Read the model definition and answer for the solid it produces. Units are mm, in the model's axes. A direction names the side the tool comes from. Round coordinates to 2 decimals unless told otherwise and drop trailing zeros. Order: outer loops, then holes, each group sorted by start corner. A loop starts at its lowest first (then second) coordinate and runs counter-clockwise, first axis right, second up. Notation, with made-up numbers: (84.25, 16) - (97.25, 16) arc R26 cw to (97.25, 34) - close; hole circle Ø10 at (11.25, 77). An arc over 180 degrees is marked (long way). One line per question, with ' | ' between items. Start each with the question number.
1) Flat-ended cylindrical pins translate along their axes: pin 1 (5 mm diameter, centred on y = 15, z = -2, fed in from +X); pin 2 (8 mm diameter, centred on x = -4.5, y = -0.5, fed in from -Z); pin 3 (0.6 mm diameter, centred on x = -2, z = 6.5, fed in from -Y); pin 4 (8 mm diameter, centred on x = 4.5, y = -18.5, fed in from +Z). Find the tip coordinate at first contact, or state that the pin passes through.
2) The part is cut by section C-C, the plane x = 9.5. Give the vertices of the cut face in (y, z).
3) The part is cut by section A-A, the plane y = 9.14. Give the vertices of the cut face in (x, z), plus the area to 3 significant figures.
4) Straight lines are drawn through the part: line 1 (X direction, y = -14.5, z = 2.5); line 2 (Z direction, x = -2, y = 9); line 3 (Y direction, x = -3.75, z = 3.25). For each, find the intervals that lie inside material, in ascending order. Write a range as from..to.
5) The part is cut by section B-B, the plane z = 2.95. Count the separate pieces of the cut face and the enclosed holes in it, plus the area to 3 significant figures.
6) For faces 1 (the flat face through (1.059, -17, -2)), 2 (the flat face through (4, 17, 5.9)), 3 (the flat face through (4, -17, 5.9)), 4 (the flat face through (3.6, 13.85, -0.6)), 5 (the flat face through (6.219, -17, -2)), determine the directions among +Z, -Z, +X, -X, +Y, -Y from which every point of the face is accessible in a straight line to the end or side of a thin tool.
7) The mould has two halves that part along X. Classify faces 6 (the flat face through (3, 13.6, 7)), 7 (the cylindrical face through (12.04, -15.8, 2.99)), 8 (the flat face through (6.219, 17, -2)), 9 (the cylindrical face through (3.58, 17.25, -0.85)): pulls with the +X half, pulls with the -X half, needs draft (parallel to the pull), parting line crosses it, or undercut.
8) The part is cut by section D-D, the plane x = 12.75. Give the vertices of the cut face in (y, z).
from build123d import *

# Parameters (mm, degrees)
F1_DEPTH = 20.75
F2_W     = 25.3
F2_H     = 27.2
F3_DEPTH = 2
F2_R     = 1.7
F4_DEPTH = 9.251
F5_W     = 27.7
F5_H     = 3.35
F5_R     = 1.21
F6_DEPTH = 25.301


with BuildPart() as f1:
    # F0 (on Front) → F1 (new body, symmetric)
    with BuildSketch(Plane.XZ):
        Polygon((16.2885056366, 5.9), (-9.0114943634, 5.9), (-9.0114943634, 0), (1.0585056366, 0), (6.2185056366, 0), (16.2885056366, 0), align=None)
        with BuildLine():
            Line((6.2185056366, 0), (1.0585056366, 0))
            Line((1.0585056366, 0), (1.0585056366, -3.35))
            Line((1.0585056366, -3.35), (1.1385056366, -3.35))
            ThreePointArc((1.1385056366, -3.35), (3.6385056366, -0.85), (6.1385056366, -3.35))
            Line((6.1385056366, -3.35), (6.2185056366, -3.35))
            Line((6.2185056366, -3.35), (6.2185056366, 0))
        make_face()
    extrude(amount=F1_DEPTH, both=True)

    # F2 (on face) → F3 (join)
    with BuildSketch(Plane.XY.offset(5.9)):
        with Locations((3.6385056366, 0)):
            Rectangle(F2_W, F2_H)
    extrude(amount=F3_DEPTH)

    # F2 (on face) → F4 (cut, through all)
    with BuildSketch(Plane.XY.offset(5.9)):
        with Locations((13.7385056366, 15.875)):
            Circle(F2_R)
        with Locations((-6.4614943634, 15.875)):
            Circle(F2_R)
        with Locations((-6.4614943634, -15.875)):
            Circle(F2_R)
        with Locations((13.7385056366, -15.875)):
            Circle(F2_R)
    extrude(amount=-F4_DEPTH, mode=Mode.SUBTRACT)

    # F5 (on face) → F6 (cut, through all)
    with BuildSketch(Plane(origin=(-9.0114943634, 0, 0), x_dir=(0, -1, 0), z_dir=(-1, 0, 0))):
        with Locations((0, -1.675)):
            Rectangle(F5_W, F5_H)
        with Locations((9.14, 2.95)):
            Circle(F5_R)
        with Locations((-9.14, 2.95)):
            Circle(F5_R)
    extrude(amount=-F6_DEPTH, mode=Mode.SUBTRACT)


solid = f1.part
Values:
1) pin 1: stops at x = 16.29 | pin 2: stops at z = 0 | pin 3: stops at y = -13.6 | pin 4: stops at z = 5.9
2) outline: (-20.75, 0) - (20.75, 0) - (20.75, 5.9) - (13.6, 5.9) - (13.6, 7.9) - (-13.6, 7.9) - (-13.6, 5.9) - (-20.75, 5.9) - close; hole circle Ø2.42 at (-9.14, 2.95); hole circle Ø2.42 at (9.14, 2.95)
3) outline: (-9.01, 0) - (16.29, 0) - (16.29, 1.74) - (-9.01, 1.74) - close; (-9.01, 4.16) - (16.29, 4.16) - (16.29, 7.9) - (-9.01, 7.9) - close | area: 139 mm^2
4) line 1: x = -9.01..-7.46, -5.46..12.74, 14.74..16.29 | line 2: z = 0..1.75, 4.15..7.9 | line 3: y = -20.75..-10.31, -7.97..7.97, 10.31..20.75
5) separate pieces: 3 | enclosed holes: 4 | area: 891 mm^2
6) face 1: -Z, -X, +Y, -Y | face 2: +Z, +X, -X, +Y | face 3: +Z, +X, -X, -Y | face 4: -Z, +X, -X | face 5: -Z, +X, +Y, -Y
7) face 6: needs draft | face 7: undercut | face 8: pulls with the +X half | face 9: undercut
8) outline: (-20.75, 0) - (-17.26, 0) - (-17.26, 5.9) - (-20.75, 5.9) - close; (-14.49, 0) - (14.49, 0) - (14.49, 5.9) - (13.6, 5.9) - (13.6, 7.9) - (-13.6, 7.9) - (-13.6, 5.9) - (-14.49, 5.9) - close; (17.26, 0) - (20.75, 0) - (20.75, 5.9) - (17.26, 5.9) - close; hole circle Ø2.42 at (-9.14, 2.95); hole circle Ø2.42 at (9.14, 2.95)
